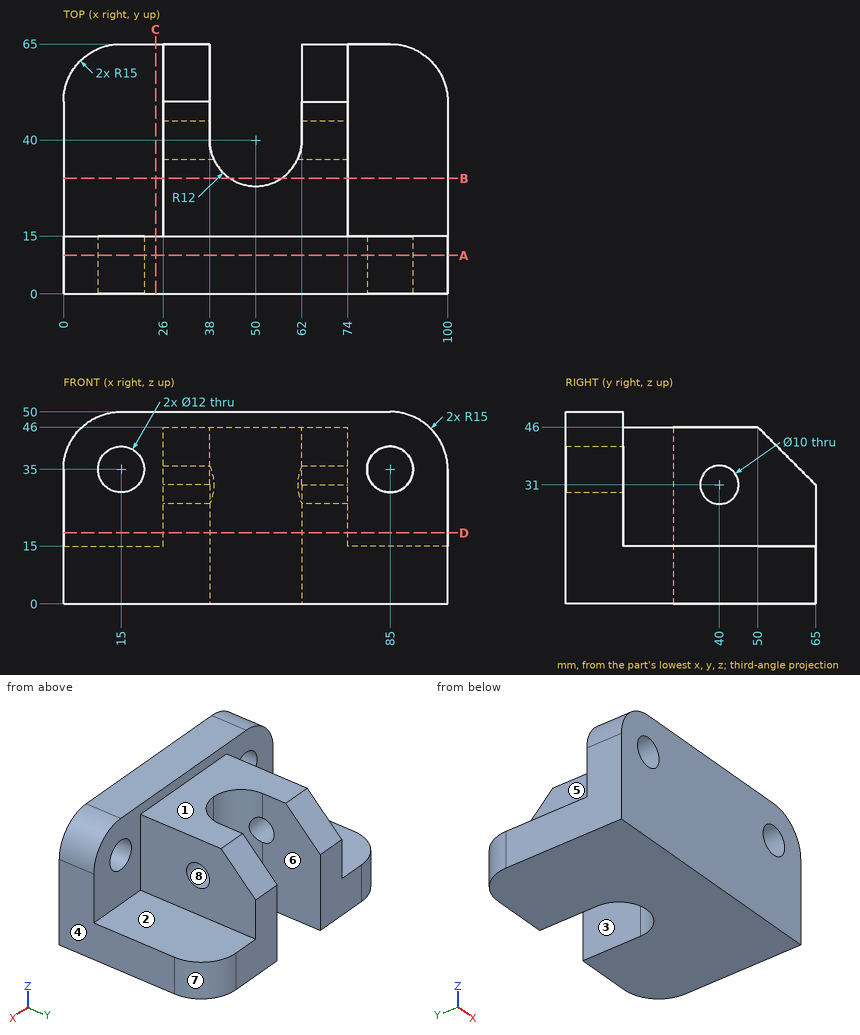
Input: dimensioned drawing with shaded views. Units: mm. Origin: part minimum x, y, z. A direction names the side the tool comes from. Give positions to 0.01 mm unless a question says otherwise; leave off trailing zeros. Write each loop counter-clockwise with the first axis right and the second up, starting at its lowest first coordinate (ties: lowest second). Pieces come first, ordered by that corner, then holes.
Q1. Section D-D, the plane z = 18.5. Output: boundary loops of the cut face in (x, y).
Q2. Pull-direction query (Y, two-part tool) for the marked faces 6, 7 and 8; classes: pulls with the +Y half, pulls with the -Y half, needs draft (parallel to the pull), parting line crosses it, or undercut.
Q3. Set-up query: the marked faces 1, 2, 3, 4 and 5. Return all of +Z, -Z, +X, -X, +Y, -Y with unobstructed straight access to the full face (end or side cutting, diameter ignored); none if empty.
Q4. Section A-A, the plane y = 10. Output: boundary loops of the cut face in (x, z), plus the area to 3 significant figures.
Q5. Section B-B, the plane y = 30. Output: boundary loops of the cut face in (x, z).
Q6. Section C-C, the plane x = 24. Output: boundary loops of the cut face in (y, z), plus the area to 3 significant figures.
Q7. First-contact query: P1, Ø1.5, axis at x = 42, z = 37, coming from the -Y side; P2, Ø7.5, axis at y = 54.5, z = 27, coming from the -X side; P3, Ø2, axis at x = 44, z = 13.5, coming from the +Y side; P4, Ø16, axis at y = 40, z = 31, coming from the +X side. Flat tips, straight axial feed; report the tip coordinate or a pass-through.
Q8. Material intervals for probe 1 along Z at (x, y) = (64.25, 40); probe 2 along X at (y, z) = (41, 45); probe 3 along Z at (x, y) = (85, 8), sorted ascending.
Filled in:
1. outline: (0, 0) - (100, 0) - (100, 15) - (74, 15) - (74, 65) - (62, 65) - (62, 40) arc R12 cw to (38, 40) - (38, 65) - (26, 65) - (26, 15) - (0, 15) - close
2. face 6: needs draft
2. face 7: pulls with the +Y half
2. face 8: undercut
3. face 1: +Z, +X, -X, +Y
3. face 2: +Z, +X, +Y
3. face 3: +Z, -Z, +Y
3. face 4: +Z, -Z, +X, +Y, -Y
3. face 5: +Z, -X, +Y
4. outline: (0, 0) - (100, 0) - (100, 35) arc R15 ccw to (85, 50) - (15, 50) arc R15 ccw to (0, 35) - close; hole circle Ø12 at (15, 35); hole circle Ø12 at (85, 35)
4. area: 4,680 mm2
5. outline: (0, 0) - (43.37, 0) - (43.37, 46) - (26, 46) - (26, 15) - (0, 15) - close; (56.63, 0) - (100, 0) - (100, 15) - (74, 15) - (74, 46) - (56.63, 46) - close
6. outline: (0, 0) - (65, 0) - (65, 15) - (15, 15) - (15, 50) - (0, 50) - close
6. area: 1,500 mm2
7. P1: stops at y = 0
7. P2: stops at x = 26
7. P3: stops at y = 30.25
7. P4: stops at x = 74
8. probe 1: z = 0 to 26, 36 to 46
8. probe 2: x = 26 to 38, 62 to 74
8. probe 3: z = 0 to 29, 41 to 50
